Verification items for this drawing (mm, ordinates from the low corner). Round coordinates to 2 decimals unless told otherwise and drop trailing zeros. Loops run counter-clockwise (first coordinate to the right, second up) from the corner with the lowest first, then second, coordinate; pieces in that order, holes last. Notation, with made-up numbers: (68.5, 51.25) - (111.5, 51.25) arc R30 ccw to (111.5, 84.25) - close; hole circle Ø11 at (62.5, -36). An arc over 180 degrees is marked (long way). Put each result on its own line as item: value. Start each with the question number.
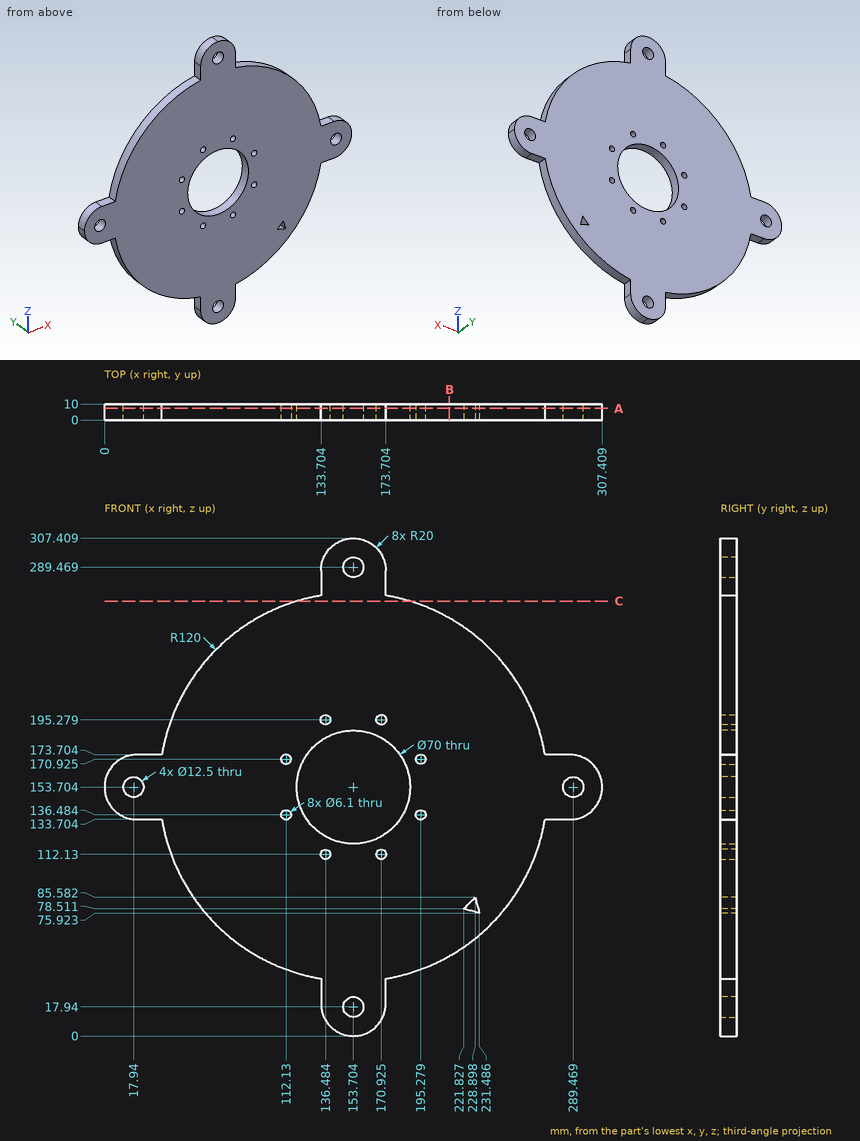
Q1. Cross-section at A-A on y = 7.25. State how many separate pieces and enclosed holes the cut face has, and give its area (3 significant figures).
Q2. Depth check by flat-ended pin: pin 1 Ø10 at (x, z) = (170.93, 195.28) entering from -Y; pin 2 Ø5 at (y, z) = (3, 279.5) entering from -X; pin 3 Ø1.5 at (x, y) = (228, 4) entering from -Z; pin 4 Ø6 at (x, y) = (46, 7) entering from -Z. Enter the tip coordinate at first touch or a pass-through.
Q3. Cross-section at C-C on z = 268.5. Enter the section's corners in (x, y).
Q4. Material ranges on line 1 (X direction, y = 7, z = 110) (1 decimal); line 2 (Z direction, x = 164, y = 6.5) (1 decimal); line 3 (Z direction, x = 14.5, y = 3.25) (1 decimal), recorded low to high. Write a range as from..to.
Q5. Cross-section at B-B on x = 213. Enter the section's corners in (y, z).
Answer list:
1. separate pieces: 1
1. enclosed holes: 14
1. area: 45,400 mm2
2. pin 1: stops at y = 0
2. pin 2: stops at x = 133.7
2. pin 3: stops at z = 58.88
2. pin 4: stops at z = 95.08
3. outline: (118.75, 0) - (188.66, 0) - (188.66, 10) - (118.75, 10) - close
4. line 1: x = 41.9..134.3, 138.7..168.7, 173.1..265.5
4. line 2: z = 2.9..120.3, 187.2..304.6
4. line 3: z = 134.5..148.5, 158.9..172.9
5. outline: (0, 49.38) - (10, 49.38) - (10, 258.03) - (0, 258.03) - close
